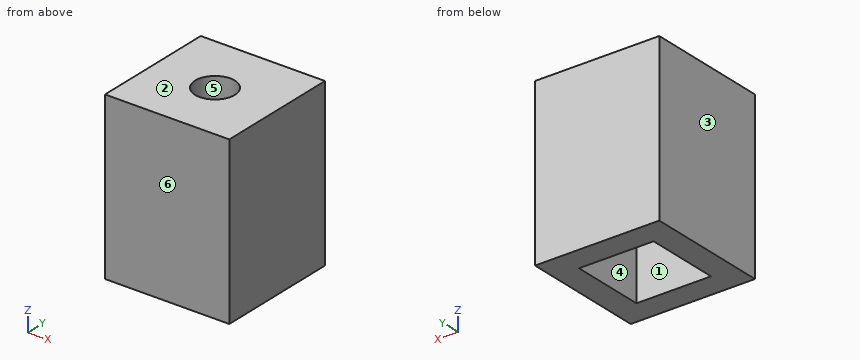
from build123d import *

# Parameters (mm, degrees)
CYLINDER111_R     = 1.2
CYLINDER111_DEPTH = 10
BOX065_W          = 4.5
BOX065_H          = 4.5
BOX065_DEPTH      = 10
BOX064_W          = 7.5
BOX064_H          = 7.5
BOX064_DEPTH      = 10


with BuildPart() as cylinder111:
    # Cylinder111 → Cylinder111 (new body)
    with BuildSketch(Plane(origin=(7.5, 16.5, 105), x_dir=(1, 0, 0), z_dir=(0, 0, 1))):
        Circle(CYLINDER111_R)
    extrude(amount=CYLINDER111_DEPTH)


with BuildPart() as cube063:
    # Box065 → Box065 (new body)
    with BuildSketch(Plane(origin=(5.25, 14.25, 98.5), x_dir=(1, 0, 0), z_dir=(0, 0, 1))):
        with Locations((2.25, 2.25)):
            Rectangle(BOX065_W, BOX065_H)
    extrude(amount=BOX065_DEPTH)


with BuildPart() as pcbmount:
    # Box064 → Box064 (new body)
    with BuildSketch(Plane(origin=(3.75, 12.75, 100), x_dir=(1, 0, 0), z_dir=(0, 0, 1))):
        with Locations((3.75, 3.75)):
            Rectangle(BOX064_W, BOX064_H)
    extrude(amount=BOX064_DEPTH)

    # Cut080: cut Cube063
    add(cube063.part, mode=Mode.SUBTRACT)

    # Cut081: cut Cylinder111
    add(cylinder111.part, mode=Mode.SUBTRACT)


with BuildPart() as pcbmount_1:
    # Cut081 placement: moved
    add(pcbmount.part.moved(Location((200, 20, -100))))


solid = pcbmount_1.part
Geometry check sheet. Reference: the model listing, model coordinates, mm. Face numbers are marked on the shaded views. A direction names the side the tool comes from. Round coordinates to 2 decimals unless told otherwise and drop trailing zeros. Write each loop counter-clockwise with the first axis right and the second up, starting at its lowest first coordinate (ties: lowest second). Pieces come first, ordered by that corner, then holes. Notation, with made-up numbers: (22.5, 40.25) -> (60.5, 40.25) arc R33 ccw to (60.5, 74.25) -> close; hole circle Ø7 at (62, 58.5). An arc over 180 degrees is marked (long way). One line per item, written item: value. Start each with the question number.
(1) Scan lines: line 1 (X direction, y = 37, z = 1.75); line 2 (X direction, y = 36.5, z = 8.9); line 3 (Y direction, x = 207.5, z = 9.45). Record each from-to range of solid material in increasing order. Write a range as [from, to].
(2) Go/stop test with a flat-tipped pin: pin 1 Ø3 at (x, y) = (207.5, 36.5) entering from -Z. Record where the tip stops, or that it passes through.
(3) Access from +Z, -Z, +X, -X, +Y, -Y to the whole of each face (thin tool, end or side, straight path). Record for the marked faces 1 and 2.
(4) Cross-section at C-C, the plane y = 36.5. Record the cut outline in (x, z), and give its area (4 significant figures).
(5) Draft check along Y on the marked faces 3, 4, 5 and 6. Enter one of: +Y half, -Y half, draft (parallel to the pull), parting line (faces both ways), or undercut.
(6) Cross-section at B-B, the plane x = 207.5. Record the cut outline in (y, z).
(7) Cross-section at D-D, the plane x = 209.5. Record the cut outline in (y, z).
(8) Cross-section at A-A, the plane z = 1. Record the cut outline in (x, y), and give its area (3 significant figures).
Answer:
1. line 1: [203.75, 205.25], [209.75, 211.25]
1. line 2: [203.75, 206.3], [208.7, 211.25]
1. line 3: [32.75, 35.3], [37.7, 40.25]
2. pin 1: z = 8.5
3. face 1: -Z
3. face 2: +Z, +X, -X, +Y, -Y
4. outline: (203.75, 0) -> (205.25, 0) -> (205.25, 8.5) -> (206.3, 8.5) -> (206.3, 10) -> (203.75, 10) -> close; (208.7, 8.5) -> (209.75, 8.5) -> (209.75, 0) -> (211.25, 0) -> (211.25, 10) -> (208.7, 10) -> close
4. area: 33.15 mm²
5. face 3: draft
5. face 4: undercut
5. face 5: undercut
5. face 6: -Y half
6. outline: (32.75, 0) -> (34.25, 0) -> (34.25, 8.5) -> (35.3, 8.5) -> (35.3, 10) -> (32.75, 10) -> close; (37.7, 8.5) -> (38.75, 8.5) -> (38.75, 0) -> (40.25, 0) -> (40.25, 10) -> (37.7, 10) -> close
7. outline: (32.75, 0) -> (34.25, 0) -> (34.25, 8.5) -> (38.75, 8.5) -> (38.75, 0) -> (40.25, 0) -> (40.25, 10) -> (32.75, 10) -> close
8. outline: (203.75, 32.75) -> (211.25, 32.75) -> (211.25, 40.25) -> (203.75, 40.25) -> close; hole (205.25, 34.25) -> (209.75, 34.25) -> (209.75, 38.75) -> (205.25, 38.75) -> close
8. area: 36.0 mm²
